Check sheet for the modelled part. Datum: model origin and axes. Units: mm. A direction names the side the tool comes from. Give positions to 0.01 mm unless a question says otherwise; leave off trailing zeros. Loops run counter-clockwise (first coordinate to the right, second up) from the corner with the lowest first, then second, coordinate; pieces in that order, holes last.
```python
from build123d import *

# Parameters (mm, degrees)
SKETCH015_W         = 30
SKETCH015_H         = 50
PAD014_DEPTH        = 5
SKETCH016_W         = 50
SKETCH016_H         = 25
PAD013_DEPTH        = 5
PAD010_DEPTH        = 3
PAD011_DEPTH        = 1.5
PAD012_DEPTH        = 3
HOLE002_D           = 4.4
HOLE002_DEPTH       = 25
HOLE002_CSINK_D     = 8
HOLE002_CSINK_ANGLE = 90
SKETCH018_W         = 40.900608
SKETCH018_H         = 56.513194
POCKET001_DEPTH     = 25
SKETCH020_W         = 45.434352
SKETCH020_H         = 34.44481
POCKET002_DEPTH     = 23.5


with BuildPart() as part:
    # Sketch015 → Pad014 (new body)
    with BuildSketch(Plane.XY):
        with Locations((15, 25)):
            Rectangle(SKETCH015_W, SKETCH015_H)
    extrude(amount=PAD014_DEPTH)

    # Sketch016 → Pad013 (join)
    with BuildSketch(Plane(origin=(0, 0, 0), x_dir=(0, -1, 0), z_dir=(-1, 0, 0))):
        with Locations((-25, 17.5)):
            Rectangle(SKETCH016_W, SKETCH016_H)
    extrude(amount=-PAD013_DEPTH)

    # Sketch014 → Pad010 (join)
    with BuildSketch(Plane.XZ):
        Polygon((5, 5), (5, 30), (30, 5), align=None)
    extrude(amount=-PAD010_DEPTH)

    # Sketch017 → Pad011 (join, symmetric)
    with BuildSketch(Plane.XZ.offset(-25)):
        Polygon((5, 5), (5, 30), (30, 5), align=None)
    extrude(amount=PAD011_DEPTH, both=True)

    # Sketch013 → Pad012 (join)
    with BuildSketch(Plane.XZ.offset(-50)):
        Polygon((5, 30), (5, 5), (30, 5), align=None)
    extrude(amount=PAD012_DEPTH)

    # Hole002
    with Locations(Plane.XY.offset(5)):
        with Locations((17.5, 36.75), (17.5, 13.25)):
            CounterSinkHole(HOLE002_D / 2, HOLE002_CSINK_D / 2, depth=HOLE002_DEPTH, counter_sink_angle=HOLE002_CSINK_ANGLE)

    # Sketch018 → Pocket001 (cut)
    with BuildSketch(Plane.XY.offset(13)):
        with Locations((14.816534, 25.266581)):
            Rectangle(SKETCH018_W, SKETCH018_H)
    extrude(amount=POCKET001_DEPTH, mode=Mode.SUBTRACT)

    # Sketch020 → Pocket002 (cut)
    with BuildSketch(Plane.XZ):
        with Locations((13.859938, 7.463043)):
            Rectangle(SKETCH020_W, SKETCH020_H)
    extrude(amount=-POCKET002_DEPTH, mode=Mode.SUBTRACT)


solid = part.part
```
(1) Gauge pin test, flat ends, axial feed: pin 1 Ø10 at (x, y) = (18, 35) entering from +Z; pin 2 Ø1.5 at (x, y) = (20, 27) entering from +Z; pin 3 Ø4 at (y, z) = (34, 10) entering from +X. Record the tip position at first contact, or that the pin passes through.
(2) Section check B-B on x = 17.5. Record the boundary of the cut face in (y, z), plus the area to 3 significant figures.
(3) Access from +Z, -Z, +X, -X, +Y, -Y to the whole of each face (thin tool, end or side, straight path). Record for faces 4 (the face through (15, 26.5, 9)), 5 (the face through (15, 37, 0)).
(4) Release check for a two-part mould opening along Y. For faces 1 (the face through (15, 50, 7)), 2 (the face through (17, 41, 5)), 3 (the face through (30, 37, 2)) record: pulls with the +Y half, pulls with the -Y half, needs draft (parallel to the pull), parting line crosses it, or undercut.
(5) Section check C-C on z = 1. Record the boundary of the cut face in (x, y).
(6) Section check A-A on y = 36.75. Record the boundary of the cut face in (x, z), plus the area to 3 significant figures.
(7) Section check D-D on x = 23. Record the boundary of the cut face in (y, z), plus the area to 4 significant figures.
(8) Material ranges on line 1 (Y direction, x = 17.5, z = 2.4); line 2 (X direction, y = 36.75, z = 2.05); line 3 (Y direction, x = 7, z = 5.75), recorded low to high.
Computed values:
1. pin 1: stops at z = 5
1. pin 2: stops at z = 13
1. pin 3: stops at x = 5
2. outline: (23.5, 0) - (34.55, 0) - (34.55, 3.2) - (32.75, 5) - (26.5, 5) - (26.5, 13) - (23.5, 13) - close; (38.95, 0) - (50, 0) - (50, 13) - (47, 13) - (47, 5) - (40.75, 5) - (38.95, 3.2) - close
2. area: 155 mm2
3. face 4: +Z, +X
3. face 5: -Z, +X, -X, +Y, -Y
4. face 1: pulls with the +Y half
4. face 2: undercut
4. face 3: needs draft
5. outline: (0, 23.5) - (30, 23.5) - (30, 50) - (0, 50) - close; hole circle Ø4.4 at (17.5, 36.75)
6. outline: (0, 0) - (15.3, 0) - (15.3, 3.2) - (13.5, 5) - (5, 5) - (5, 13) - (0, 13) - close; (19.7, 0) - (30, 0) - (30, 5) - (21.5, 5) - (19.7, 3.2) - close
6. area: 165 mm2
7. outline: (23.5, 0) - (50, 0) - (50, 12) - (47, 12) - (47, 5) - (26.5, 5) - (26.5, 12) - (23.5, 12) - close
7. area: 174.5 mm2
8. line 1: y = 23.5 to 34.55, 38.95 to 50
8. line 2: x = 0 to 15.3, 19.7 to 30
8. line 3: y = 23.5 to 26.5, 47 to 50
